CAD build for the part. Positions are in the model's coordinates, mm. Round coordinates to 2 decimals unless told otherwise and drop trailing zeros. Loops run counter-clockwise (first coordinate to the right, second up) from the corner with the lowest first, then second, coordinate; pieces in that order, holes last. Notation, with made-up numbers: M 57.25,64.5 L 71.25,64.5 A26 ccw 71.25,95.5 Z; hole C 69,78 d6. An arc over 180 degrees is marked long. Use a Markdown table: item, result. Add a question column.
(1) Band-saw the part on C-C, the plane x = 1.6. Give the number of separate pieces and of enclosed holes in the cut face, and give its area (3 significant figures).
(2) Band-saw the part on D-D, the plane y = 10.5. Write the cut outline in (x, z), and give its area (3 significant figures).
(3) Band-saw the part on A-A, the plane y = 15.5. Write the cut outline in (x, z), and give its area (3 significant figures).
(4) Flat gauge pins, fed straight in: P1, Ø4, axis at y = -5.5, z = -14, coming from the -X side; P2, Ø1.5, axis at x = 0.5, y = -8.5, coming from the +Z side. Where does each tip first touch, or does it go through?
(5) Wall check: L1, parallel to Z at x = 1.95, y = 4.5; L2, parallel to Y at x = 2.7, z = 9.5; L3, parallel to Z at x = 0.6, y = 3. Give the ranges that are in metal, low to high.
(6) Band-saw the part on B-B, the plane z = -15.5. Write the cut outline in (x, y).
(7) Two-plate mould, pull along Z, no slides. Class faces 1 (the face through (3, 0, -5)), 2 (the face through (1.521, 9.285, 17.243)): released by +Z, released by -Z, zero draft, split by the parting line, or undercut.
from build123d import *

# Parameters (mm, degrees)
SKETCH1_R           = 24
BOSS_EXTRUDE1_DEPTH = 3
SKETCH2_R           = 2
CUT_EXTRUDE1_DEPTH  = 3
CUT_EXTRUDE2_DEPTH  = 3
CIRPATTERN1_COUNT   = 10
CUT_EXTRUDE4_DEPTH  = 3


with BuildPart() as part:
    # Sketch1 → Boss-Extrude1 (new body)
    with BuildSketch(Plane(origin=(0, 0, 0), x_dir=(0, 0, -1), z_dir=(1, 0, 0))):
        Circle(SKETCH1_R)
    extrude(amount=BOSS_EXTRUDE1_DEPTH)

    # Sketch2 → Cut-Extrude1 (cut)
    with BuildSketch(Plane(origin=(3, 0, 0), x_dir=(0, 0, -1), z_dir=(1, 0, 0))):
        Circle(SKETCH2_R)
    extrude(amount=-CUT_EXTRUDE1_DEPTH, mode=Mode.SUBTRACT)

    # Sketch3 → Cut-Extrude2 (cut)
    with BuildSketch(Plane(origin=(3, 0, 0), x_dir=(0, 0, -1), z_dir=(1, 0, 0))):
        with BuildLine():
            Line((0.482962913, 6.80244213), (3.614211274, 18.488420103))
            ThreePointArc((3.614211274, 18.488420103), (3.495889099, 19.277869009), (2.837448694, 19.729184801))
            ThreePointArc((2.837448694, 19.729184801), (0, 20), (-2.837448694, 19.729184801))
            ThreePointArc((-2.837448694, 19.729184801), (-3.495889099, 19.277869009), (-3.614211274, 18.488420103))
            Line((-3.614211274, 18.488420103), (-0.482962913, 6.80244213))
            ThreePointArc((-0.482962913, 6.80244213), (0, 6.431851653), (0.482962913, 6.80244213))
        make_face()
    cut_extrude2 = extrude(amount=-CUT_EXTRUDE2_DEPTH, mode=Mode.SUBTRACT)

    # CirPattern1: Cut-Extrude2 ×10 about axis
    cirpattern1_axis = Axis((0, 0, 0), (1, 0, 0))
    for i in range(1, CIRPATTERN1_COUNT):
        add(cut_extrude2.rotate(cirpattern1_axis, i * 360 / CIRPATTERN1_COUNT), mode=Mode.SUBTRACT)

    # Sketch5 → Cut-Extrude4 (cut)
    with BuildSketch(Plane(origin=(3, 0, 0), x_dir=(0, 0, -1), z_dir=(1, 0, 0))):
        with BuildLine():
            Line((-2.109857815, 0.81), (-0.81, 0.81))
            Line((-0.81, 0.81), (-0.81, 2.109857815))
            add(Edge.make_bspline(
                [(-0.81, 2.109857815), (0, 2.410142185), (0.81, 2.109857815)],
                knots=[0, 0, 0, 1, 1, 1], degree=2))
            Line((0.81, 2.109857815), (0.81, 0.81))
            Line((0.81, 0.81), (2.109857815, 0.81))
            add(Edge.make_bspline(
                [(2.109857815, 0.81), (2.410142185, 0), (2.109857815, -0.81)],
                knots=[0, 0, 0, 1, 1, 1], degree=2))
            Line((2.109857815, -0.81), (0.81, -0.81))
            Line((0.81, -0.81), (0.81, -2.109857815))
            add(Edge.make_bspline(
                [(0.81, -2.109857815), (0, -2.410142185), (-0.81, -2.109857815)],
                knots=[0, 0, 0, 1, 1, 1], degree=2))
            Line((-0.81, -2.109857815), (-0.81, -0.81))
            Line((-0.81, -0.81), (-2.109857815, -0.81))
            add(Edge.make_bspline(
                [(-2.109857815, -0.81), (-2.410142185, 0), (-2.109857815, 0.81)],
                knots=[0, 0, 0, 1, 1, 1], degree=2))
        make_face()
    extrude(amount=-CUT_EXTRUDE4_DEPTH, mode=Mode.SUBTRACT)


solid = part.part
Return value:
| question | item | result |
|---|---|---|
| 1 | separate pieces | 1 |
| 1 | enclosed holes | 11 |
| 1 | area | 1,220 mm^2 |
| 2 | outline | M 0,-21.58 L 3,-21.58 L 3,-10.91 L 0,-10.91 Z; M 0,-5.42 L 3,-5.42 L 3,-1.47 L 0,-1.47 Z; M 0,1.47 L 3,1.47 L 3,5.42 L 0,5.42 Z; M 0,10.91 L 3,10.91 L 3,21.58 L 0,21.58 Z |
| 2 | area | 87.7 mm^2 |
| 3 | outline | M 0,-18.32 L 3,-18.32 L 3,-12.62 L 0,-12.62 Z; M 0,-7.34 L 3,-7.34 L 3,-2.81 L 0,-2.81 Z; M 0,2.81 L 3,2.81 L 3,7.34 L 0,7.34 Z; M 0,12.62 L 3,12.62 L 3,18.32 L 0,18.32 Z |
| 3 | area | 61.3 mm^2 |
| 4 | P1 | x = 0 |
| 4 | P2 | z = 22.71 |
| 5 | L1 | -23.57 to -19.46, -9.31 to 9.31, 19.46 to 23.57 |
| 5 | L2 | -22.04 to -17.53, -9.36 to -4.63, -1.79 to 1.79, 4.63 to 9.36, 17.53 to 22.04 |
| 5 | L3 | -23.81 to -19.61, -7 to 7, 19.61 to 23.81 |
| 6 | outline | M 0,-18.32 L 3,-18.32 L 3,-8.52 L 0,-8.52 Z; M 0,-2.11 L 3,-2.11 L 3,2.11 L 0,2.11 Z; M 0,8.52 L 3,8.52 L 3,18.32 L 0,18.32 Z |
| 7 | face 1 | zero draft |
| 7 | face 2 | undercut |
